Answer from the drawing. Dimensions are ordinates in mm from the lowest x, y and z of the part. Coordinates: 2 decimals unless noted, no trailing zeros. Write each loop counter-clockwise with the first axis right and the second up, starting at its lowest first coordinate (ties: lowest second). Pieces come first, ordered by that corner, then holes. Notation, with made-up numbers: (54, -23.5) -> (70, -23.5) arc R32 ccw to (70, 7.5) -> close; hole circle Ø1 at (28.25, 63). An arc over 180 degrees is marked (long way). Return JSON: item names as keys, results as strings.
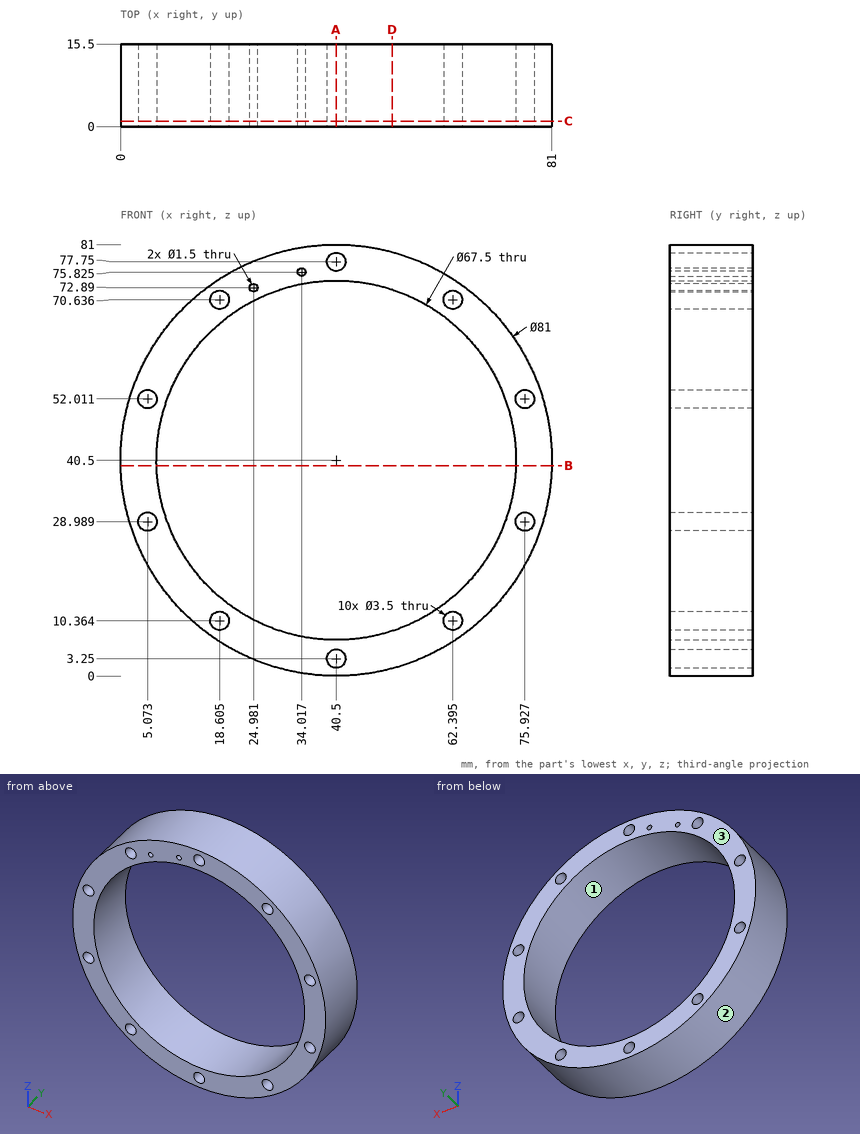
1. The part is cut by section C-C (y = 1). Count the separate pieces of the cut face and the enclosed holes in it.
Taken from the geometry:
{"separate pieces": "1", "enclosed holes": "13"}
2. For a pull along X with two mould halves and no side action, classify the marked faces 1, 2 and 3 as +X half, -X half, draft (parallel to the pull), parting line (faces both ways), or undercut.
Taken from the geometry:
{"face 1": "undercut", "face 2": "parting line", "face 3": "draft"}
3. The part is cut by section D-D (x = 51). Determine the outline of the cut face in (y, z) (1 decimal).
Taken from the geometry:
{"outline": "(0, 1.4) -> (15.5, 1.4) -> (15.5, 8.4) -> (0, 8.4) -> close; (0, 72.6) -> (15.5, 72.6) -> (15.5, 79.6) -> (0, 79.6) -> close"}
4. The part is cut by section A-A (x = 40.5). Determine the outline of the cut face in (y, z), then the cut area to 3 significant figures.
Taken from the geometry:
{"outline": "(0, 0) -> (15.5, 0) -> (15.5, 1.5) -> (0, 1.5) -> close; (0, 5) -> (15.5, 5) -> (15.5, 6.75) -> (0, 6.75) -> close; (0, 74.25) -> (15.5, 74.25) -> (15.5, 76) -> (0, 76) -> close; (0, 79.5) -> (15.5, 79.5) -> (15.5, 81) -> (0, 81) -> close", "area": "101 mm2"}
5. The part is cut by section B-B (z = 39.5). Determine the outline of the cut face in (x, y) (1 decimal), then the cut area to 3 significant figures.
Taken from the geometry:
{"outline": "(0, 0) -> (6.8, 0) -> (6.8, 15.5) -> (0, 15.5) -> close; (74.2, 0) -> (81, 0) -> (81, 15.5) -> (74.2, 15.5) -> close", "area": "209 mm2"}
6. Consider L1, parallel to Z at x = 74.5, y = 2 (1 decimal); L2, parallel to X at y = 2, z = 51.5; L3, parallel to X at y = 9, z = 19 (1 decimal). Determine where each line is inside the solid, lowest interval first.
Taken from the geometry:
{"L1": "z = 18.5 to 28, 30 to 51, 53 to 62.5", "L2": "x = 1.52 to 3.4, 6.75 to 8.59, 72.41 to 74.25, 77.6 to 79.48", "L3": "x = 6.2 to 14.5, 66.5 to 74.8"}
7. Flat-ended cylindrical pins translate along their axes: pin 1 Ø1.5 at (y, z) = (5.5, 37) entering from -X; pin 2 Ø4 at (y, z) = (5, 44) entering from -X; pin 3 Ø3 at (x, z) = (75.93, 28.99) entering from +Y; pin 4 Ø1 at (x, y) = (45.5, 6.5) entering from +Z. Find the tip coordinate at first contact, or state that the pin passes through.
Taken from the geometry:
{"pin 1": "stops at x = 0.09", "pin 2": "stops at x = 0.03", "pin 3": "passes through", "pin 4": "stops at z = 80.75"}
